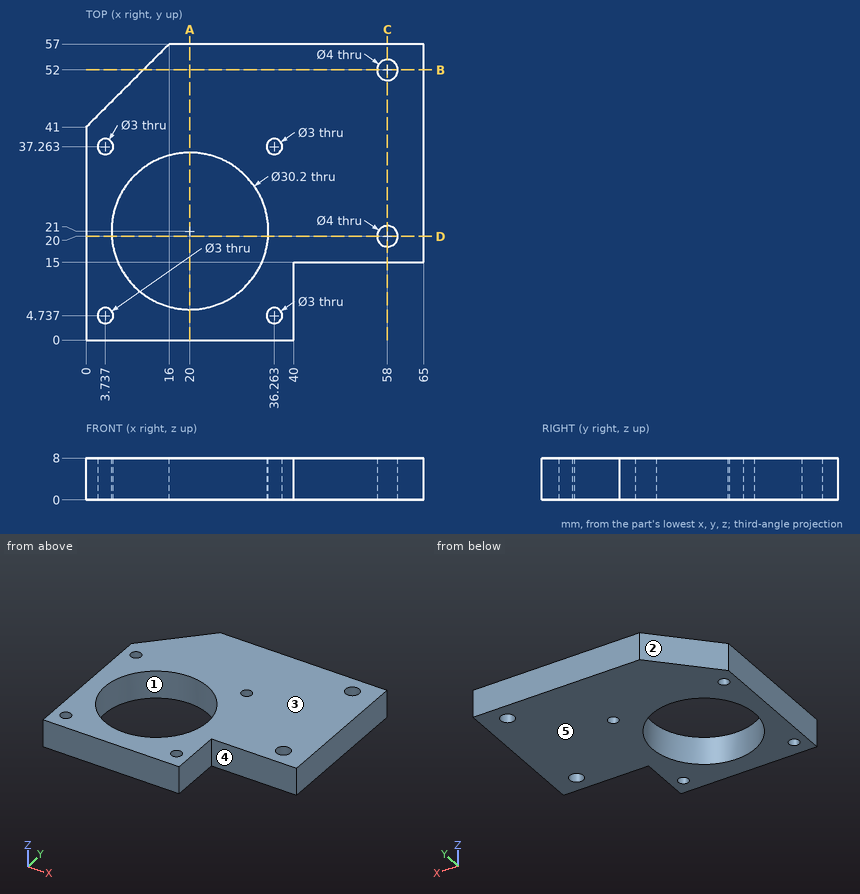
Verification items for this drawing (mm, ordinates from the low corner). A direction names the side the tool comes from. Coordinates: 2 decimals unless noted, no trailing zeros. Order: outer loops, then holes, each group sorted by start corner. A loop starts at its lowest first (then second) coordinate and runs counter-clockwise, first axis right, second up. Notation, with made-up numbers: (6.25, 2.25) -> (50.25, 2.25) arc R25 cw to (50.25, 29.25) -> close; hole circle Ø11 at (35.25, 25). An arc over 180 degrees is marked (long way). Put each result on its own line as item: value. Start each with the question number.
1. Cross-section at B-B, the plane y = 52. Record the boundary of the cut face in (x, z).
2. Access from +Z, -Z, +X, -X, +Y, -Y to the whole of each face (thin tool, end or side, straight path). Record for the marked faces 4 and 5.
3. Cross-section at C-C, the plane x = 58. Record the boundary of the cut face in (y, z).
4. Go/stop test with a flat-tipped pin: pin 1 Ø2.5 at (x, z) = (57.5, 5.5) entering from -Y. Record where the tip stops, or that it passes through.
5. Cross-section at D-D, the plane y = 20. Record the boundary of the cut face in (x, z), then the cut area to 3 significant figures.
6. Cross-section at A-A, the plane x = 20. Record the boundary of the cut face in (y, z).
7. Material ranges on L1, parallel to Y at x = 58, z = 5.75; L2, parallel to Y at x = 20, z = 4.25; L3, parallel to Y at x = 36, z = 5.5, recorded low to high. Write a range as [from, to].
8. Mould release check, pull along Y, two halves, no side actions. Record for the marked faces 1, 2 and 3: released by +Y, released by -Y, zero draft, split by the parting line, or undercut.
Computed:
1. outline: (11, 0) -> (56, 0) -> (56, 8) -> (11, 8) -> close; (60, 0) -> (65, 0) -> (65, 8) -> (60, 8) -> close
2. face 4: +Z, -Z, +X, -Y
2. face 5: -Z, +X, -X, +Y, -Y
3. outline: (15, 0) -> (18, 0) -> (18, 8) -> (15, 8) -> close; (22, 0) -> (50, 0) -> (50, 8) -> (22, 8) -> close; (54, 0) -> (57, 0) -> (57, 8) -> (54, 8) -> close
4. pin 1: y = 15
5. outline: (0, 0) -> (4.93, 0) -> (4.93, 8) -> (0, 8) -> close; (35.07, 0) -> (56, 0) -> (56, 8) -> (35.07, 8) -> close; (60, 0) -> (65, 0) -> (65, 8) -> (60, 8) -> close
5. area: 247 mm2
6. outline: (0, 0) -> (5.9, 0) -> (5.9, 8) -> (0, 8) -> close; (36.1, 0) -> (57, 0) -> (57, 8) -> (36.1, 8) -> close
7. L1: [15, 18], [22, 50], [54, 57]
7. L2: [0, 5.9], [36.1, 57]
7. L3: [0, 3.26], [6.21, 35.79], [38.74, 57]
8. face 1: undercut
8. face 2: released by +Y
8. face 3: zero draft
